from build123d import *

# Parameters (mm, degrees)
F0_W     = 50
F0_H     = 50
F1_DEPTH = 10
F3_DEPTH = 25
F5_D     = 12
F5_DEPTH = 5
F5_TIP   = 3.6051637142


with BuildPart() as f1:
    # F0 (on Top) → F1 (new body)
    with BuildSketch(Plane.XY):
        Rectangle(F0_W, F0_H)
    extrude(amount=F1_DEPTH)

    # F2 (on Right) → F3 (join, symmetric)
    with BuildSketch(Plane.YZ):
        Polygon((0, -10), (0, 0), (-7.9979246179, 0), (-15, -10), align=None)
        Polygon((7.9979246179, 0), (0, 0), (0, -10), (15, -10), align=None)
    extrude(amount=F3_DEPTH, both=True)

    # F5
    with Locations(Plane(origin=(0, 0, -10), x_dir=(1, 0, 0), z_dir=(0, 0, -1))):
        with Locations((0, 0)):
            Hole(F5_D / 2, depth=F5_DEPTH)
            with Locations((0, 0, -(F5_DEPTH + F5_TIP / 2))):  # 118° drill point
                Cone(0, F5_D / 2, F5_TIP, mode=Mode.SUBTRACT)


solid = f1.part
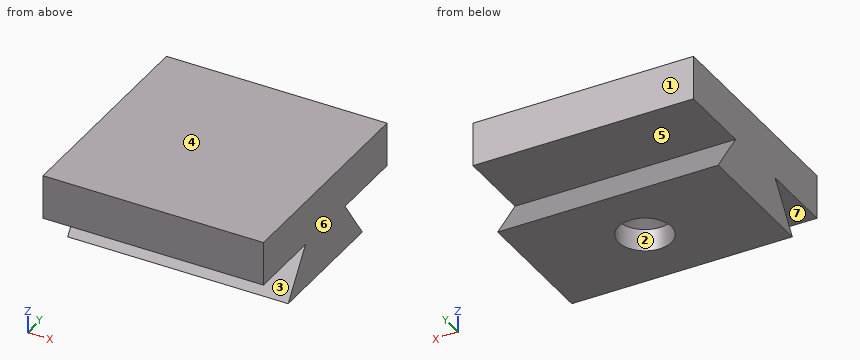
Geometry check sheet. Reference: the model listing, model coordinates, mm. Face numbers are marked on the shaded views. A direction names the side the tool comes from. Give positions to 0.01 mm unless a question says otherwise; leave off trailing zeros. Write each loop counter-clockwise with the first axis right and the second up, starting at its lowest first coordinate (ties: lowest second). Pieces come first, ordered by that corner, then holes.
1) Thickness scan on line 1 (Z direction, x = -8, y = -11.5); line 2 (Z direction, x = 2, y = -12.5); line 3 (Z direction, x = -21, y = 17). Record the ranges inside material, lowest first.
Values follow:
line 1: z = -10 to -5, 0 to 10
line 2: z = -10 to -6.43, 0 to 10
line 3: z = 0 to 10
2) Cross-section at C-C (z = -5.75). Record the boundary of the cut face in (x, y), plus the area to 3 significant figures.
Values follow:
outline: (-25, -12.02) - (25, -12.02) - (25, 12.02) - (-25, 12.02) - close; hole circle Ø12 at (0, 0)
area: 1,090 mm2
3) Set-up check for the marked faces 5, 6 and 7: record each of +Z, -Z, +X, -X, +Y, -Y from which the full face is reachable in a straight line by a thin tool's end or side.
Values follow:
face 5: +X, -X, +Y
face 6: +Z, -Z, +X, +Y, -Y
face 7: +X, -X, -Y
4) Cross-section at A-A (y = 12). Record the boundary of the cut face in (x, z).
Values follow:
outline: (-25, -10) - (25, -10) - (25, -5.72) - (-25, -5.72) - close; (-25, 0) - (25, 0) - (25, 10) - (-25, 10) - close
5) Cross-section at B-B (x = 7.5). Record the boundary of the cut face in (y, z), plus the area to 3 significant figures.
Values follow:
outline: (-25, 0) - (-8, 0) - (-15, -10) - (15, -10) - (8, 0) - (25, 0) - (25, 10) - (-25, 10) - close
area: 730 mm2
6) Go/stop test with flat-tipped pins: pin 1 Ø5 at (y, z) = (13.5, -5) entering from -X; pin 2 Ø11 at (x, y) = (0, 0) entering from -Z. Record where each tip stops, or that it passes through.
Values follow:
pin 1: stops at x = -25
pin 2: stops at z = -4.7
7) Cross-section at D-D (z = -2.75). Record the boundary of the cut face in (x, y).
Values follow:
outline: (-25, -9.92) - (25, -9.92) - (25, 9.92) - (-25, 9.92) - close; hole circle Ø4.51 at (0, 0)
8) Release check for a two-part mould opening along Y. For the marked faces 1, 2, 3 and 4 record: released by +Y, released by -Y, zero draft, split by the parting line, or undercut.
Values follow:
face 1: released by +Y
face 2: undercut
face 3: released by -Y
face 4: zero draft
